from build123d import *

# Parameters (mm, degrees)
ESTRUSIONE_ESTRUSIONE1_DEPTH = 57
SCHIZZO2_R                   = 1.5
TAGLIO_ESTRUSIONE1_DEPTH     = 57
SMUSSO1_SIZE                 = 7


with BuildPart() as part:
    # Schizzo1 → Estrusione-Estrusione1 (new body)
    with BuildSketch(Plane.XY):
        Polygon((0, 0), (20, 0), (20, 23), (45, 23), (45, 26), (17, 26), (17, 3), (-5, 3), (-5, 0), align=None)
    extrude(amount=ESTRUSIONE_ESTRUSIONE1_DEPTH)

    # Schizzo2 → Taglio-Estrusione1 (cut)
    with BuildSketch(Plane(origin=(0, 3, 0), x_dir=(1, 0, 0), z_dir=(0, 1, 0))):
        with Locations(Location((0, -50.5, 0), (0, 0, 270))):
            Circle(SCHIZZO2_R)
        with Locations(Location((0, -6.5, 0), (0, 0, 270))):
            Circle(SCHIZZO2_R)
    extrude(amount=-TAGLIO_ESTRUSIONE1_DEPTH, mode=Mode.SUBTRACT)

    # Smusso1
    smusso1_edges = [part.edges().sort_by_distance(p)[0] for p in [
        (-5, 1.5, 57),
        (-5, 1.5, 0),
    ]]
    chamfer(smusso1_edges, length=SMUSSO1_SIZE)


solid = part.part
The model under review builds one solid part; all positions refer to its coordinate system, in mm. A direction names the side the tool comes from. Give positions to 0.01 mm unless a question says otherwise; leave off trailing zeros. Loops run counter-clockwise (first coordinate to the right, second up) from the corner with the lowest first, then second, coordinate; pieces in that order, holes last. Notation, with made-up numbers: (-25, 19) -> (-20, 19) arc R34 cw to (-20, 53) -> close; hole circle Ø2 at (26, -40). An arc over 180 degrees is marked (long way). Answer as a JSON object with one key per item and string values. Group by question number.
Q1. Take a section at A-A (x = 0). Write out the cut boundary in (y, z).
Q2. Draft analysis for pull direction Z (two halves, no side actions). For faces 1 (the flat face through (31, 26, 28)), 2 (the flat face through (19, 15, 0)), 3 (the flat face through (19, 15, 57)), 4 (the cylindrical face through (0, 2, 49)), state which applies: pulls with the +Z half, pulls with the -Z half, needs draft (parallel to the pull), parting line crosses it, or undercut.
Q3. Take a section at D-D (z = 53). Write out the cut boundary in (x, y), plus the area to 3 significant figures.
Q4. Take a section at B-B (z = 11). Write out the cut boundary in (x, y), plus the area to 3 significant figures.
Q5. Take a section at C-C (y = 23.75). Write out the cut boundary in (x, z).
Q6. Tool access review of faces 5 (the flat face through (20, 11, 28)), 6 (the flat face through (-2, 2, 53)), 7 (the flat face through (17, 15, 28)): name each direction out of +Z, -Z, +X, -X, +Y, -Y from which nothing blocks a thin tool from reaching the whole face with its end or side.
Q7. Insertion check: pin 1 (10 mm diameter, centred on x = 28.5, z = 20.5, fed in from -Y); pin 2 (2 mm diameter, centred on y = 8.5, z = 40.5, fed in from -X); pin 3 (11 mm diameter, centred on x = 5, z = 26, fed in from +Y). Each pin has a flat end and moves straight along its axis. Give the tip position at first contact, or say it passes through.
Q8. Wall thickness on line 1 along Y through (x, z) = (2.5, 27); line 2 along X through (y, z) = (19.25, 23.5); line 3 along Y through (x, z) = (40, 49.5): over which ranges is each line inside the solid? List them lowest first.
Answer below:
{
 "1": {"outline": "(0, 2) -> (3, 2) -> (3, 5) -> (0, 5) -> close; (0, 8) -> (3, 8) -> (3, 49) -> (0, 49) -> close; (0, 52) -> (3, 52) -> (3, 55) -> (0, 55) -> close"},
 "2": {"face 1": "needs draft", "face 2": "pulls with the -Z half", "face 3": "pulls with the +Z half", "face 4": "undercut"},
 "3": {"outline": "(-2, 0) -> (20, 0) -> (20, 23) -> (45, 23) -> (45, 26) -> (17, 26) -> (17, 3) -> (-2, 3) -> close", "area": "210 mm2"},
 "4": {"outline": "(-5, 0) -> (20, 0) -> (20, 23) -> (45, 23) -> (45, 26) -> (17, 26) -> (17, 3) -> (-5, 3) -> close", "area": "219 mm2"},
 "5": {"outline": "(17, 0) -> (45, 0) -> (45, 57) -> (17, 57) -> close"},
 "6": {"face 5": "+Z, -Z, +X, -Y", "face 6": "+Z, -X, +Y, -Y", "face 7": "+Z, -Z, -X, +Y"},
 "7": {"pin 1": "stops at y = 23", "pin 2": "stops at x = 17", "pin 3": "stops at y = 3"},
 "8": {"line 1": "y = 0 to 3", "line 2": "x = 17 to 20", "line 3": "y = 23 to 26"}
}
